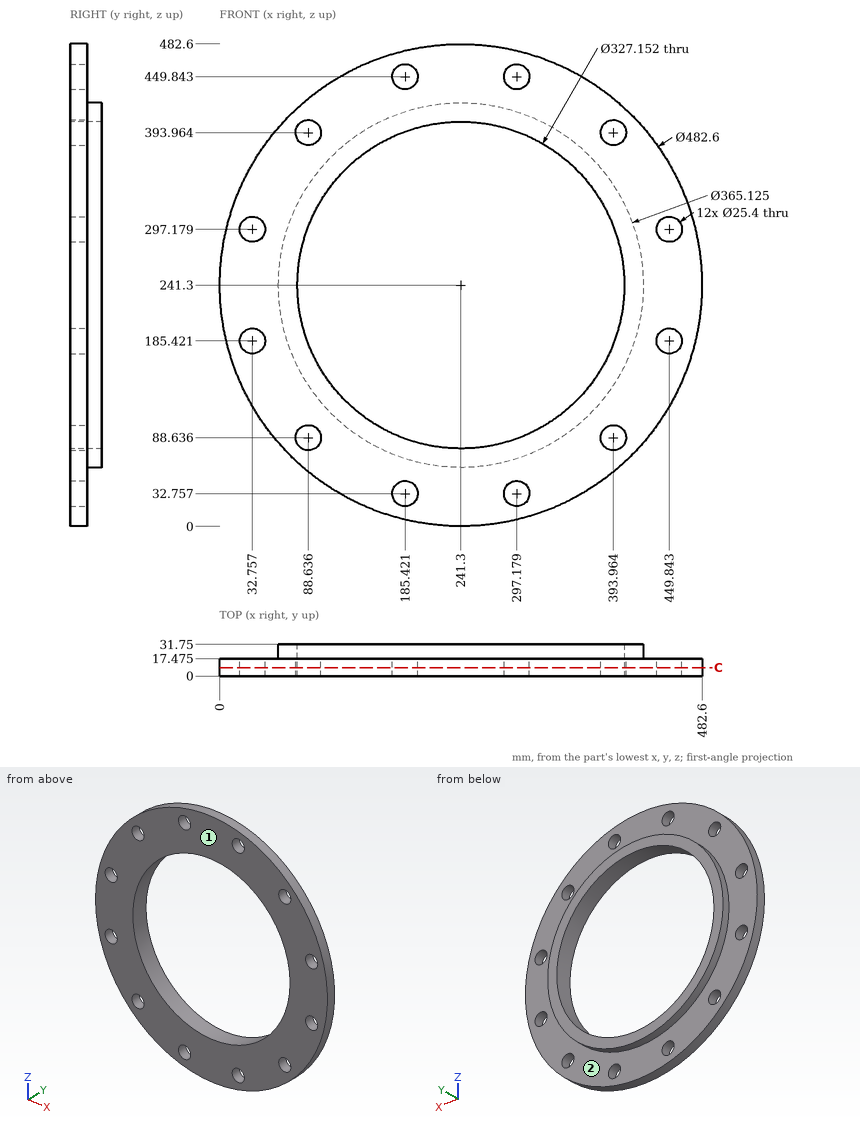
Check sheet for the drawn part. Datum: minimum x, y, z corner. Units: mm. A direction names the side the tool comes from. Coordinates: 2 decimals unless noted, no trailing zeros. Return JSON: item names as keys, results as strings.
(1) Go/stop test with flat-tipped pins: pin 1 (5 mm diameter, centred on y = 14, z = 339.5, fed in from -X); pin 2 (6 mm diameter, centred on y = 10, z = 286, fed in from -X); pin 3 (6 mm diameter, centred on x = 82, z = 225, fed in from -Y); pin 4 (1.5 mm diameter, centred on y = 4.5, z = 88, fed in from +X). Record where each tip stops, or that it passes through.
Filled sheet:
{"pin 1": "stops at x = 19.79", "pin 2": "stops at x = 3.63", "pin 3": "passes through", "pin 4": "stops at x = 428.26"}
(2) Section check C-C, the plane y = 8.5. Give the number of separate pieces and of enclosed holes in the cut face, and give its area (3 significant figures).
Filled sheet:
{"separate pieces": "1", "enclosed holes": "13", "area": "92,800 mm^2"}
(3) Access from +Z, -Z, +X, -X, +Y, -Y to the whole of each face (thin tool, end or side, straight path). Record for the marked faces 1 and 2.
Filled sheet:
{"face 1": "+Z, -Z, +X, -X, -Y", "face 2": "+Y"}
(4) Thickness scan on line 1 along Z through (x, y) = (258.5, 30); line 2 along X through (y, z) = (29, 378) (1 decimal); line 3 along X through (y, z) = (9, 273.5) (1 decimal). Record the ranges inside material, lowest first.
Filled sheet:
{"line 1": "z = 59.55 to 78.63, 403.97 to 423.05", "line 2": "x = 120.3 to 151.5, 331.1 to 362.3", "line 3": "x = 2.2 to 80.9, 401.7 to 480.4"}
